Check sheet for the modelled part. Datum: model origin and axes. Units: mm. A direction names the side the tool comes from. Round coordinates to 2 decimals unless told otherwise and drop trailing zeros. Order: outer loops, then holes, each group sorted by start corner. A loop starts at its lowest first (then second) coordinate and runs counter-clockwise, first axis right, second up.
(1) Sectioned sample at B-B, the plane z = 43.5. Enter the section's corners in (x, y), and give its area (3 significant figures).
(2) Depth check by flat-ended pin: pin 1 (4 mm diameter, centred on y = 10, z = 70.5, fed in from -X); pin 2 (8 mm diameter, centred on y = -4, z = 39, fed in from +X); pin 3 (4.5 mm diameter, centred on x = 0, y = 50, fed in from -Z); pin 4 (4.5 mm diameter, centred on x = 0, z = 20, fed in from -Y). Enter the tip coordinate at first touch or a pass-through.
(3) Thickness scan on probe 1 along Y at (x, z) = (0, 46); probe 2 along Y at (x, z) = (0, 169); probe 3 along X at (y, z) = (35, 20). Record the ranges inside material, lowest first.
(4) Sectioned sample at C-C, the plane x = 0. Count the separate pieces of the cut face and the enclosed holes in it, and give its area (3 significant figures).
(5) Sectioned sample at D-D, the plane z = 152.5. Enter the section's corners in (x, y), and give its area (3 significant figures).
(6) Tool access check on faces 4 (the cylindrical face through (-11.923, -3.755, 70.507)), 5 (the cylindrical face through (-0.54, 47.56, 57.89)), 6 (the flat face through (11, 11, 72)). Record the directions out of +Z, -Z, +X, -X, +Y, -Y that give a thin tool (end or side, any length) a straight path to the whole face; none if there is none.
(7) Sectioned sample at A-A, the plane y = 0. Enter the section's corners in (x, z).
(8) Mould release check, pull along Y, two halves, no side actions. Record for faces 1 (the cylindrical face through (-0.33, 32.33, 97.48)), 2 (the flat face through (-24, 8, 0)), 3 (the flat face through (5.9, -11.5, 70)): released by +Y, released by -Y, zero draft, split by the parting line, or undercut.
```python
from build123d import *

# Parameters (mm, degrees)
F3_R      = 3.5
F5_R      = 2.5
F7_R      = 25
F8_DEPTH  = 138
F9_R      = 25
F10_DEPTH = 70


with BuildPart() as f1:
    # F0 (on Front) → F1 (revolve)
    with BuildSketch(Plane.XZ):
        Polygon((-25, 210), (-27, 210), (-27, 0), (-25, 0), (-25, 70), (-12.5, 70), (-12.5, 71), (-13.5, 72), (-25, 72), align=None)
    revolve(axis=Axis((0, 0, 105), (0, 0, 1)))

    # F4: sweep along a path in F2
    with BuildLine(Plane.YZ) as f4_path:
        Line((0, 20), (40, 20))
        ThreePointArc((40, 20), (47.0710678119, 22.9289321881), (50, 30))
        Line((50, 30), (50, 85))
        ThreePointArc((50, 85), (47.0710678119, 92.0710678119), (40, 95))
        Line((40, 95), (0, 95))
    # F3 (on Front) → F4 (sweep)
    with BuildSketch(Plane.XZ):
        with Locations((0, 20)):
            Circle(F3_R)
    sweep(path=f4_path.line)

    # F6: sweep along a path in F2
    with BuildLine(Plane.YZ) as f6_path:
        Line((0, 20), (40, 20))
        ThreePointArc((40, 20), (47.0710678119, 22.9289321881), (50, 30))
        Line((50, 30), (50, 85))
        ThreePointArc((50, 85), (47.0710678119, 92.0710678119), (40, 95))
        Line((40, 95), (0, 95))
    # F5 (on Front) → F6 (sweep, cut)
    with BuildSketch(Plane.XZ):
        with Locations((0, 20)):
            Circle(F5_R)
    sweep(path=f6_path.line, mode=Mode.SUBTRACT)

    # F7 (on face) → F8 (cut, through all)
    with BuildSketch(Plane.XY.offset(210)):
        Circle(F7_R)
    extrude(amount=-F8_DEPTH, mode=Mode.SUBTRACT)

    # F9 (on face) → F10 (cut, through all)
    with BuildSketch(Plane(origin=(0, 0, 0), x_dir=(1, 0, 0), z_dir=(0, 0, -1))):
        Circle(F9_R)
    extrude(amount=-F10_DEPTH, mode=Mode.SUBTRACT)


solid = f1.part
```
Derived:
1. outline: circle Ø54 at (0, 0); circle Ø7 at (0, 50); hole circle Ø50 at (0, 0); hole circle Ø5 at (0, 50)
1. area: 346 mm2
2. pin 1: stops at x = -25.79
2. pin 2: stops at x = 27
2. pin 3: stops at z = 18.95
2. pin 4: stops at y = -27
3. probe 1: y = -27 to -25, 25 to 27, 46.5 to 47.5, 52.5 to 53.5
3. probe 2: y = -27 to -25, 25 to 27
3. probe 3: x = -3.5 to -2.5, 2.5 to 3.5
4. separate pieces: 3
4. enclosed holes: 1
4. area: 1,090 mm2
5. outline: circle Ø54 at (0, 0); hole circle Ø50 at (0, 0)
5. area: 327 mm2
6. face 4: +Z, -Z
6. face 5: none
6. face 6: +Z
7. outline: (-27, 0) - (-25, 0) - (-25, 70) - (-12.5, 70) - (-12.5, 71) - (-13.5, 72) - (-25, 72) - (-25, 210) - (-27, 210) - close; (12.5, 70) - (25, 70) - (25, 0) - (27, 0) - (27, 210) - (25, 210) - (25, 72) - (13.5, 72) - (12.5, 71) - close
8. face 1: undercut
8. face 2: zero draft
8. face 3: undercut
